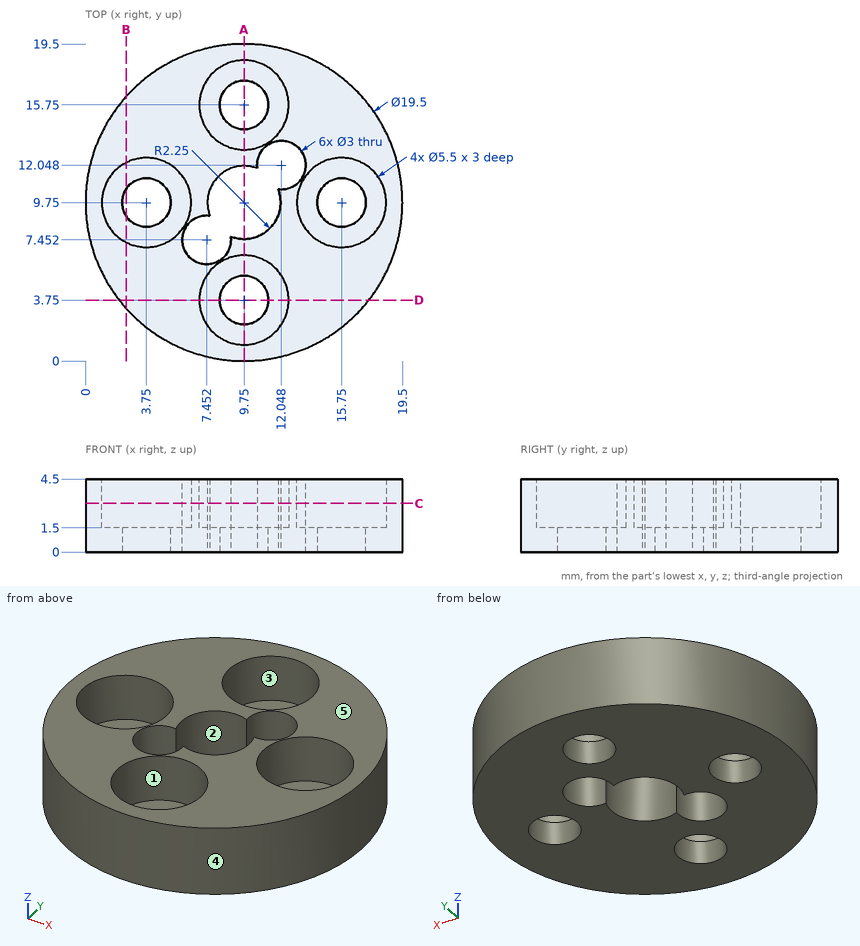
Verification items for this drawing (mm, ordinates from the low corner). A direction names the side the tool comes from. Round coordinates to 2 decimals unless told otherwise and drop trailing zeros. Write each loop counter-clockwise with the first axis right and the second up, starting at its lowest first coordinate (ties: lowest second). Pieces come first, ordered by that corner, then holes. Notation, with made-up numbers: (-13, -37) - (46, -37) arc R31 cw to (46, -12) - close; hole circle Ø2 at (81, 21.25). An arc over 180 degrees is marked (long way). Answer as a JSON object with one key per item and string values. Group by question number.
Q1. Section check C-C, the plane z = 3. Enter the section's corners in (x, y), plus the area to 3 significant figures.
Q2. Go/stop test with flat-tipped pins: pin 1 Ø4 at (x, y) = (15.75, 9.75) entering from +Z; pin 2 Ø1.5 at (y, z) = (11, 3) entering from -X; pin 3 Ø2 at (x, z) = (17, 1) entering from -Y. Record where each tip stops, or that it passes through.
Q3. Mould release check, pull along X, two halves, no side actions. Record for the marked faces 3, 4 and 5: released by +X, released by -X, zero draft, split by the parting line, or undercut.
Q4. Tool access check on the marked faces 1 and 2. Record the directions out of +Z, -Z, +X, -X, +Y, -Y that give a thin tool (end or side, any length) a straight path to the whole face; none if there is none.
Q5. Section check A-A, the plane x = 9.75. Enter the section's corners in (y, z), plus the area to 3 significant figures.
Q6. Section check D-D, the plane y = 3.75. Enter the section's corners in (x, z), plus the area to 3 significant figures.
Q7. Thickness scan on line 1 (Y direction, x = 9.75, z = 0.35); line 2 (X direction, y = 8.5, z = 1.7); line 3 (Y direction, x = 11.5, z = 2.7) (1 decimal). Record the ranges inside material, lowest first.
Q8. Section check B-B, the plane x = 2.5. Enter the section's corners in (y, z), plus the area to 3 significant figures.
Found:
{
 "1": {"outline": "circle Ø19.5 at (9.75, 9.75); hole circle Ø5.5 at (3.75, 9.75); hole circle Ø5.5 at (9.75, 3.75); hole circle Ø5.5 at (9.75, 15.75); hole (7.65, 8.94) arc R1.5 ccw (long way) to (8.94, 7.65) arc R2.25 ccw to (11.85, 10.56) arc R1.5 ccw (long way) to (10.56, 11.85) arc R2.25 ccw to start; hole circle Ø5.5 at (15.75, 9.75)", "area": "175 mm^2"},
 "2": {"pin 1": "stops at z = 1.5", "pin 2": "stops at x = 0.01", "pin 3": "stops at y = 2.27"},
 "3": {"face 3": "undercut", "face 4": "split by the parting line", "face 5": "zero draft"},
 "4": {"face 1": "+Z", "face 2": "+Z, -Z"},
 "5": {"outline": "(0, 0) - (2.25, 0) - (2.25, 1.5) - (1, 1.5) - (1, 4.5) - (0, 4.5) - close; (5.25, 0) - (7.5, 0) - (7.5, 4.5) - (6.5, 4.5) - (6.5, 1.5) - (5.25, 1.5) - close; (12, 0) - (14.25, 0) - (14.25, 1.5) - (13, 1.5) - (13, 4.5) - (12, 4.5) - close; (17.25, 0) - (19.5, 0) - (19.5, 4.5) - (18.5, 4.5) - (18.5, 1.5) - (17.25, 1.5) - close", "area": "25.5 mm^2"},
 "6": {"outline": "(2.06, 0) - (8.25, 0) - (8.25, 1.5) - (7, 1.5) - (7, 4.5) - (2.06, 4.5) - close; (11.25, 0) - (17.44, 0) - (17.44, 4.5) - (12.5, 4.5) - (12.5, 1.5) - (11.25, 1.5) - close", "area": "48.2 mm^2"},
 "7": {"line 1": "y = 0 to 2.25, 5.25 to 7.5, 12 to 14.25, 17.25 to 19.5", "line 2": "x = 0.08 to 1.3, 6.2 to 6.38, 11.62 to 13.3, 18.2 to 19.42", "line 3": "y = 0.2 to 1.6, 5.9 to 8.3, 13.4 to 13.6, 17.9 to 19.3"},
 "8": {"outline": "(3.23, 0) - (8.92, 0) - (8.92, 1.5) - (7.3, 1.5) - (7.3, 4.5) - (3.23, 4.5) - close; (10.58, 0) - (16.27, 0) - (16.27, 4.5) - (12.2, 4.5) - (12.2, 1.5) - (10.58, 1.5) - close", "area": "41.5 mm^2"}
}
